Work out the finished part from the listing and answer in its coordinate system (mm). A direction names the side the tool comes from. Round coordinates to 2 decimals unless told otherwise and drop trailing zeros. Loops run counter-clockwise (first coordinate to the right, second up) from the corner with the lowest first, then second, coordinate; pieces in that order, holes last.
from build123d import *

# Parameters (mm, degrees)
BOSS_EXTRUDE1_DEPTH = 100
SKETCH2_R           = 1.75
CUT_EXTRUDE1_DEPTH  = 113.585800614
CUT_EXTRUDE2_DEPTH  = 8.25


with BuildPart() as part:
    # Sketch1 → Boss-Extrude1 (new body)
    with BuildSketch(Plane.XY):
        with BuildLine():
            Line((50, 10.224622738), (50, 5.224622738))
            ThreePointArc((50, 5.224622738), (45, 3.884876776), (41.339745962, 0.224622738))
            ThreePointArc((41.339745962, 0.224622738), (38.927083678, -2.096523604), (35.710580838, -3.025377262))
            Line((35.710580838, -3.025377262), (14.289419162, -3.025377262))
            ThreePointArc((14.289419162, -3.025377262), (11.039419162, -2.154542386), (8.660254038, 0.224622738))
            ThreePointArc((8.660254038, 0.224622738), (5, 3.884876776), (0, 5.224622738))
            Line((0, 5.224622738), (0, 10.224622738))
            Line((0, 10.224622738), (14.25, 10.224622738))
            Line((14.25, 10.224622738), (14.25, 3.724622738))
            ThreePointArc((14.25, 3.724622738), (14.762563133, 2.487185871), (16, 1.974622738))
            Line((16, 1.974622738), (34, 1.974622738))
            ThreePointArc((34, 1.974622738), (35.237436867, 2.487185871), (35.75, 3.724622738))
            Line((35.75, 3.724622738), (35.75, 10.224622738))
            Line((35.75, 10.224622738), (50, 10.224622738))
        make_face()
    extrude(amount=-BOSS_EXTRUDE1_DEPTH)

    # Sketch2 → Cut-Extrude1 (cut, through all)
    with BuildSketch(Plane.XZ.offset(3.025377262)):
        with Locations(Location((44.756824718, -26.634894448, 0), (0, 0, 270))):
            Circle(SKETCH2_R)
        with Locations(Location((44.756824718, -4.537105649, 0), (0, 0, 270))):
            Circle(SKETCH2_R)
        with Locations(Location((44.756824718, -71.972969116, 0), (0, 0, 270))):
            Circle(SKETCH2_R)
        with Locations(Location((44.756824718, -94.070757915, 0), (0, 0, 270))):
            Circle(SKETCH2_R)
        with Locations(Location((5.243175282, -71.972969116, 0), (0, 0, 270))):
            Circle(SKETCH2_R)
        with Locations(Location((5.243175282, -94.070757915, 0), (0, 0, 270))):
            Circle(SKETCH2_R)
        with Locations(Location((5.243175282, -26.634894448, 0), (0, 0, 270))):
            Circle(SKETCH2_R)
        with Locations(Location((5.243175282, -4.537105649, 0), (0, 0, 270))):
            Circle(SKETCH2_R)
    extrude(amount=-CUT_EXTRUDE1_DEPTH, mode=Mode.SUBTRACT)

    # Sketch3 → Cut-Extrude2 (cut)
    with BuildSketch(Plane.XZ.offset(3.025377262)):
        Polygon((8.243175282, -2.805054841), (5.243175282, -1.073004033), (2.243175282, -2.805054841), (2.243175282, -6.269156456), (5.243175282, -8.001207264), (8.243175282, -6.269156456), align=None)
        Polygon((5.264020111, -23.170855549), (2.25365201, -24.884822847), (2.232807181, -28.348861746), (5.222330453, -30.098933346), (8.232698554, -28.384966048), (8.253543382, -24.920927149), align=None)
        Polygon((41.746456618, -24.920927149), (44.735979889, -23.170855549), (47.74634799, -24.884822847), (47.767192819, -28.348861746), (44.777669547, -30.098933346), (41.767301446, -28.384966048), align=None)
        Polygon((41.756824718, -6.269156456), (41.756824718, -2.805054841), (44.756824718, -1.073004033), (47.756824718, -2.805054841), (47.756824718, -6.269156456), (44.756824718, -8.001207264), align=None)
        Polygon((41.756824718, -92.338707108), (44.756824718, -90.6066563), (47.756824718, -92.338707108), (47.756824718, -95.802808723), (44.756824718, -97.534859531), (41.756824718, -95.802808723), align=None)
        Polygon((5.251618805, -68.508877791), (2.247405955, -70.233611149), (2.238962432, -73.697702473), (5.234731759, -75.437060441), (8.238944609, -73.712327084), (8.247388132, -70.248235759), align=None)
        Polygon((5.243175282, -90.6066563), (2.243175282, -92.338707108), (2.243175282, -95.802808723), (5.243175282, -97.534859531), (8.243175282, -95.802808723), (8.243175282, -92.338707108), align=None)
        Polygon((41.752611868, -70.248235759), (44.748381195, -68.508877791), (47.752594045, -70.233611149), (47.761037568, -73.697702473), (44.765268241, -75.437060441), (41.761055391, -73.712327084), align=None)
    extrude(amount=-CUT_EXTRUDE2_DEPTH, mode=Mode.SUBTRACT)


solid = part.part
Item 1: Section A-A, the plane y = 7 is taken. State how many separate pieces and enclosed holes the cut face has, plus the area to 3 significant figures.
Item 2: Each of these flat-tipped pins is pushed along its axis until it touches: P1, Ø5, axis at x = 45.5, z = -26, coming from the -Y side; P2, Ø3, axis at x = 6.5, z = -5, coming from the -Y side; P3, Ø1.7, axis at y = 4, z = -93, coming from the -X side; P4, Ø3, axis at x = 5.24, z = -71.97, coming from the -Y side (1 decimal). Where does it stop, or does it pass through?
Item 3: For faces 1 (the face through (35.22, 2.47, -49.3)), 2 (the face through (42.9, 3.51, -91.68)), 3 (the face through (5.77, 7.69, -73.64)), determine the directions among +Z, -Z, +X, -X, +Y, -Y from which every point of the face is accessible in a straight line to the end or side of a thin tool.
Item 4: Section D-D, the plane y = -1.25 is taken. Give the vertices of the cut face in (x, z).
Item 5: Straight lines are drawn through the part: line 1 (X direction, y = 8.25, z = -24.5); line 2 (Y direction, x = 27.5, z = -82.5); line 3 (X direction, y = 1.5, z = -24.5). For each, find the intervals that lie inside material, in ascending order.
Item 6: Section C-C, the plane x = 22 is taken. Give the vertices of the cut face in (y, z), plus the area to 3 significant figures.
Item 7: Determine the mould class of faces 4 (the face through (45.94, 4.8, -7.32)), 5 (the face through (43, 10.225, -49)) for opening direction Z: pulls with the +Z half, pulls with the -Z half, needs draft (parallel to the pull), parting line crosses it, or undercut.
Item 8: Section B-B, the plane z = -89 is taken. Give the vertices of the cut face in (x, y).
Answer below:
1. separate pieces: 2
1. enclosed holes: 8
1. area: 2,770 mm2
2. P1: stops at y = 4.06
2. P2: stops at y = 5.22
2. P3: stops at x = 7.92
2. P4: passes through
3. face 1: +Z, -Z, +Y
3. face 2: -Y
3. face 3: +Y, -Y
4. outline: (9.83, -100) - (40.09, -100) - (40.09, 0) - (9.83, 0) - close
5. line 1: x = 0 to 14.25, 35.75 to 50
5. line 2: y = -3.03 to 1.97
5. line 3: x = 7.79 to 42.21
6. outline: (-3.03, -100) - (1.97, -100) - (1.97, 0) - (-3.03, 0) - close
6. area: 500 mm2
7. face 4: undercut
7. face 5: needs draft
8. outline: (0, 5.22) arc R10 cw to (8.66, 0.22) arc R6.5 ccw to (14.29, -3.03) - (35.71, -3.03) arc R6.97 ccw to (41.34, 0.22) arc R10 cw to (50, 5.22) - (50, 10.22) - (35.75, 10.22) - (35.75, 3.72) arc R1.75 cw to (34, 1.97) - (16, 1.97) arc R1.75 cw to (14.25, 3.72) - (14.25, 10.22) - (0, 10.22) - close
